Design review of the part built by this model. Coordinates are the model's own, in mm. Coordinates: 2 decimals unless noted, no trailing zeros. Order: outer loops, then holes, each group sorted by start corner. A loop starts at its lowest first (then second) coordinate and runs counter-clockwise, first axis right, second up. Notation, with made-up numbers: (32.25, -28) - (43.25, -28) arc R4 ccw to (43.25, -24) - close; hole circle Ø9 at (6.25, -24.75). An arc over 180 degrees is marked (long way). Write item = value, one per line. Start each with the question number.
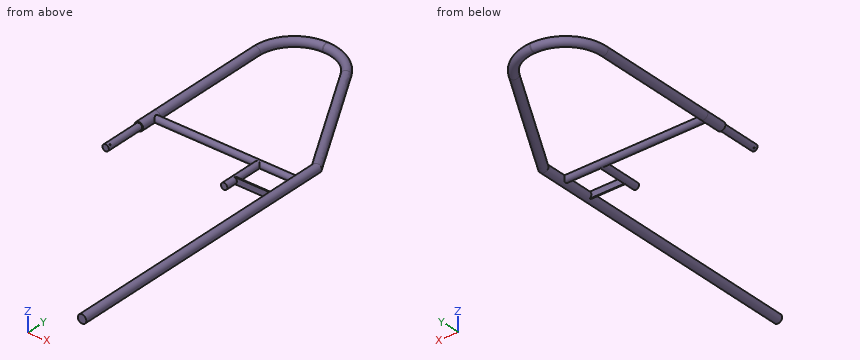
Autodesk Inventor part; units mm, degrees
ref_plane "YZ Plane" through (0, 0, 0) normal (1, 0, 0) x (0, 1, 0)
ref_plane "XY Plane" through (0, 0, 0) normal (0, 0, 1) x (1, 0, 0)
ref_plane "Arbeitsebene3" through (-18.0987, -249.8051, 17.2464) normal (-0.7239, 0, 0.6899) x (0, -1, 0)
sketch "Skizze1" plane through (0, 0, 0) normal (0, 1, 0) x (-1, 0, 0)
  circle A0 centre (0, 0) radius 20
  dimension "d0" = 40
sketch "Skizze2" plane through (0, 0, 0) normal (0, 0, 1) x (1, 0, 0)
  line L0 (0, 0) -> (0, 570)
  line L1 (180, 750) -> (183.4788, 750)
  line L2 (356.6838, 650) -> (680, 90)
  line L3 (680, 90) -> (680, -1250)
  arc A0 (180, 750) -> (0, 570) centre (180, 570) ccw
  arc A1 (356.6838, 650) -> (183.4788, 750) centre (183.4788, 550) ccw
  point P0 (0, 750)
  dimension "d1" = 750
  dimension "d4" = 90
  dimension "d8" = 2000
  dimension "d9" = 30
  dimension "d10" = 680
  dimension "d11" = 180
  dimension "d12" = 200
sweep "Sweeping1" add profiles "Skizze1" path "Skizze2"
sketch "Skizze3" plane through (0, 0, 0) normal (1, 0, 0) x (0, 1, 0)
  circle A0 centre (-20, 0) radius 15
  line L0 (0, 20) -> (0, -20)
  point P0 (0, 0)
  point P1 (0, 0)
  dimension "d16" = 30
  dimension "d27" = 20
extrude "Extrusion1" add sketch "Skizze3" along normal blind 680
sketch "Skizze4" plane through (0, 0, 0) normal (0, -1, 0) x (1, 0, 0)
  circle A0 centre (0, 0) radius 20
extrude "Extrusion2" add sketch "Skizze4" along normal blind 100
ref_plane "Arbeitsebene1" through (0, -20, 0) normal (0, 1, 0) x (-1, 0, 0)
sketch "Skizze5" plane through (0, -20, 0) normal (0, 1, 0) x (-1, 0, 0)
  circle A0 centre (0, 0) radius 20
  circle A1 centre (-500, 0) radius 15
  dimension "d23" = 30
  dimension "d24" = 500
extrude "Extrusion3" add sketch "Skizze5" against normal blind 200 contours A1
ref_plane "Arbeitsebene2" through (500, -160, 0) normal (0, -1, 0) x (1, 0, 0)
sketch "Skizze6" plane through (500, -160, 0) normal (0, -1, 0) x (1, 0, 0)
  circle A0 centre (180, 0) radius 20
  circle A1 centre (0, 0) radius 15
  line L0 (0, 15) -> (180, 15)
  line L1 (180, 15) -> (180, -15)
  line L2 (180, -15) -> (0, -15)
  line L3 (0, -15) -> (0, 15)
  point P0 (-500, 0)
  dimension "d29" = 30
  dimension "d30" = 15
  dimension "d31" = 0
extrude "Extrusion4" add sketch "Skizze6" along normal blind 5 contours L0 L1 L2 A0 | A0 L2 A1 L0 | A1 L3 picked at (173.3822, 0.8057) picked at (4.2301, 4.0345)
sketch "Skizze7" plane through (0, -100, 0) normal (0, -1, 0) x (1, 0, 0)
  circle A0 centre (0, 0) radius 20
  circle A1 centre (0, 0) radius 15
  dimension "d34" = 30
extrude "Extrusion5" add sketch "Skizze7" along normal blind 190 contours A1
ref_plane "Arbeitsebene4" through (0, -100, 0) normal (-0.6899, 0, -0.7239) x (0, -1, 0)
ref_plane "Arbeitsebene3" through (-18.0987, -249.8051, 17.2464) normal (-0.7239, 0, 0.6899) x (0, -1, 0)
sketch "Skizze8" plane through (0, -100, 0) normal (-0.6899, 0, -0.7239) x (0, -1, 0)
  line L0 (190, -15) -> (190, 15)
  line L1 (0, 15) -> (0, -15)
  point P0 (-100, 0)
  point P1 (176.4483, 0)
hole "Bohrung1" at (0, -276.4483, 0) direction (0.6899, 0, 0.7239) diameter 5 end through all both
properties part number "Geländer kurz"
Item 1: For P1, Ø9, axis at x = 604.5, z = 3.5, coming from the +Y side; P2, Ø10, axis at x = 180, z = 10, coming from the +Y side; P3, Ø9, axis at x = -3, z = -3.5, coming from the -Y side, all flat-tipped, find the tip position at first contact; note any pin that passes through.
Item 2: Add section C-C on y = -486. Give the boundary of the cut face in (x, z), plus the area to 3 significant figures.
Item 3: For line 1 (X direction, y = -140, z = 10.5); line 2 (Y direction, x = 357.5, z = 1); line 3 (Y direction, x = 170, z = -4.5), list the stretches that pass through material, from the lowest coordinate up.
Item 4: Add section B-B on z = 0. State how many separate pieces and enclosed holes the cut face has, plus the area to 3 significant figures.
Item 5: Add section A-A on y = -183.5. Give the boundary of the cut face in (x, z).
Worked out:
q1.P1 = 268.08
q1.P2 = 769.36
q1.P3 = -290
q2.outline = circle Ø40 at (680, 0)
q2.area = 1,260 mm2
q3.line_1 = -10.71 to 10.71, 489.29 to 510.71, 662.98 to 697.02
q3.line_2 = -34.97 to -5.03, 608.64 to 684.56
q3.line_3 = -34.31 to -5.69, 730.2 to 769.24
q4.separate_pieces = 1
q4.enclosed_holes = 3
q4.area = 157,000 mm2
q5.outline = circle Ø30 at (0, 0); circle Ø30 at (500, 0); circle Ø40 at (680, 0)
